Geometry check sheet. Reference: drawing and pictorial views, mm from the part's lowest x, y, z. A direction names the side the tool comes from. Give positions to 0.01 mm unless a question says otherwise; leave off trailing zeros. Write each loop counter-clockwise with the first axis right and the second up, starting at its lowest first coordinate (ties: lowest second). Pieces come first, ordered by that corner, then holes.
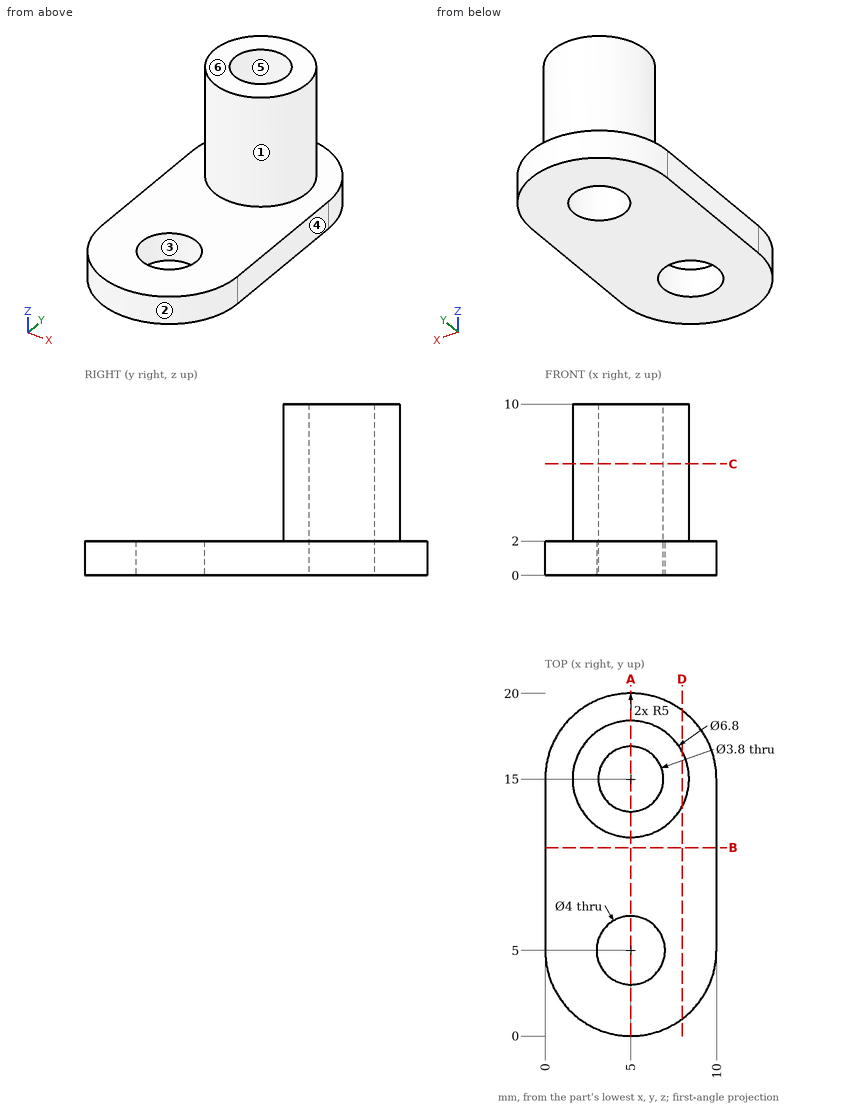
Item 1: Sectioned sample at C-C on z = 6.5. Record the cut outline in (x, y), then the cut area to 3 significant figures.
Answer key:
outline: circle Ø6.8 at (5, 15); hole circle Ø3.8 at (5, 15)
area: 25.0 mm2
Item 2: Scan lines: line 1 along Y through (x, z) = (5, 0.4); line 2 along Y through (x, z) = (5, 7.75); line 3 along Y through (x, z) = (6.25, 0.75). Record each from-to range of solid material in increasing order.
Answer key:
line 1: y = 0 to 3, 7 to 13.1, 16.9 to 20
line 2: y = 11.6 to 13.1, 16.9 to 18.4
line 3: y = 0.16 to 3.44, 6.56 to 13.57, 16.43 to 19.84
Item 3: Sectioned sample at B-B on y = 11. Record the cut outline in (x, z), then the cut area to 3 significant figures.
Answer key:
outline: (0, 0) - (10, 0) - (10, 2) - (0, 2) - close
area: 20.0 mm2
Item 4: Release check for a two-part mould opening along X. For the marked faces 3, 4, 5 and 6 record: released by +X, released by -X, zero draft, split by the parting line, or undercut.
Answer key:
face 3: undercut
face 4: released by +X
face 5: undercut
face 6: zero draft
Item 5: Sectioned sample at A-A on x = 5. Record the cut outline in (y, z), then the cut area to 3 significant figures.
Answer key:
outline: (0, 0) - (3, 0) - (3, 2) - (0, 2) - close; (7, 0) - (13.1, 0) - (13.1, 10) - (11.6, 10) - (11.6, 2) - (7, 2) - close; (16.9, 0) - (20, 0) - (20, 2) - (18.4, 2) - (18.4, 10) - (16.9, 10) - close
area: 48.4 mm2
Item 6: Sectioned sample at D-D on x = 8. Record the cut outline in (y, z), then the cut area to 3 significant figures.
Answer key:
outline: (1, 0) - (19, 0) - (19, 2) - (16.6, 2) - (16.6, 10) - (13.4, 10) - (13.4, 2) - (1, 2) - close
area: 61.6 mm2
Item 7: Set-up check for the marked faces 1 and 2: record each of +Z, -Z, +X, -X, +Y, -Y from which the full face is reachable in a straight line by a thin tool's end or side.
Answer key:
face 1: +Z
face 2: +Z, -Z, -Y
Item 8: Depth check by flat-ended pin: pin 1 (3 mm diameter, centred on y = 17.5, z = 6.5, fed in from +X); pin 2 (4 mm diameter, centred on y = 11.5, z = 8, fed in from -X); pin 3 (4 mm diameter, centred on x = 1.5, y = 4.5, fed in from +Z). Enter the tip coordinate at first touch or a pass-through.
Answer key:
pin 1: stops at x = 8.25
pin 2: stops at x = 1.95
pin 3: stops at z = 2
